```python
from build123d import *

# Parameters (mm, degrees)
SKETCH1_R             = 97.5
BOSS_EXTRUDE1_DEPTH   = 15
SKETCH2_R             = 27.5
CUT_EXTRUDE1_DEPTH    = 139.699315067
SKETCH3_R             = 3.589640567
CUT_EXTRUDE2_DEPTH    = 9.646154
CIRPATTERN1_START     = 5.353845626
CIRPATTERN1_OUTLINE_R = 3.589640567
CIRPATTERN1_DEPTH     = 9.646154374


# Read off the part's stored shape, not the designer's step: CirPattern1
with BuildPart() as part:
    # Sketch1 → Boss-Extrude1 (new body)
    with BuildSketch(Plane(origin=(0, 0, 0), x_dir=(1, 0, 0), z_dir=(0, 1, 0))):
        with Locations(Location((0, 0, 0), (0, 0, 270))):
            Circle(SKETCH1_R)
    extrude(amount=BOSS_EXTRUDE1_DEPTH)

    # Sketch2 → Cut-Extrude1 (cut, through all)
    with BuildSketch(Plane(origin=(0, 0, 0), x_dir=(1, 0, 0), z_dir=(0, 1, 0))):
        with Locations(Location((0, 0, 0), (0, 0, 270))):
            Circle(SKETCH2_R)
    extrude(amount=CUT_EXTRUDE1_DEPTH, mode=Mode.SUBTRACT)

    # Sketch3 → Cut-Extrude2 (cut)
    with BuildSketch(Plane(origin=(0, 15, 0), x_dir=(1, 0, 0), z_dir=(0, 1, 0))):
        with Locations(Location((-40.912084687, 0, 0), (0, 0, 270))):
            Circle(SKETCH3_R)
    extrude(amount=-CUT_EXTRUDE2_DEPTH, mode=Mode.SUBTRACT)

    # CirPattern1 outline → CirPattern1 (cut)
    with BuildSketch(Plane(origin=(0, 0, 0), x_dir=(1, 0, 0), z_dir=(0, 1, 0)).offset(CIRPATTERN1_START)):
        with Locations((0, 40.912084687)):
            Circle(CIRPATTERN1_OUTLINE_R)
        with Locations((40.912084687, 0)):
            Circle(CIRPATTERN1_OUTLINE_R)
        with Locations((0, -40.912084687)):
            Circle(CIRPATTERN1_OUTLINE_R)
    extrude(amount=CIRPATTERN1_DEPTH, mode=Mode.SUBTRACT)


solid = part.part
```
Check sheet for the modelled part. Datum: model origin and axes. Units: mm. A direction names the side the tool comes from. Give positions to 0.01 mm unless a question says otherwise; leave off trailing zeros. Order: outer loops, then holes, each group sorted by start corner. A loop starts at its lowest first (then second) coordinate and runs counter-clockwise, first axis right, second up. Notation, with made-up numbers: (49, 44.5) -> (76, 44.5) arc R23 cw to (76, 76.5) -> close; hole circle Ø4 at (-8.75, 62.25). An arc over 180 degrees is marked (long way). Return JSON: item names as keys, results as strings.
1. Mould release check, pull along Z, two halves, no side actions. Record for faces 3 (the cylindrical face through (-86.5, 7.4, 44.99)), 4 (the flat face through (-20, 15, 20)), 5 (the flat face through (-41, 5.354, 0)): +Z half, -Z half, draft (parallel to the pull), parting line (faces both ways), or undercut.
From the geometry:
{"face 3": "parting line", "face 4": "draft", "face 5": "undercut"}
2. Cross-section at C-C, the plane z = 52.5. Record the cut outline in (x, y), plus the area to 3 significant figures.
From the geometry:
{"outline": "(-82.16, 0) -> (82.16, 0) -> (82.16, 15) -> (-82.16, 15) -> close", "area": "2,460 mm^2"}
3. Cross-section at A-A, the plane x = 0. Record the cut outline in (y, z).
From the geometry:
{"outline": "(0, -97.5) -> (15, -97.5) -> (15, -44.5) -> (5.35, -44.5) -> (5.35, -37.32) -> (15, -37.32) -> (15, -27.5) -> (0, -27.5) -> close; (0, 27.5) -> (15, 27.5) -> (15, 37.32) -> (5.35, 37.32) -> (5.35, 44.5) -> (15, 44.5) -> (15, 97.5) -> (0, 97.5) -> close"}
4. Cross-section at B-B, the plane y = 11.75. Record the cut outline in (x, z).
From the geometry:
{"outline": "circle Ø195 at (0, 0); hole circle Ø7.18 at (-40.91, 0); hole circle Ø55 at (0, 0); hole circle Ø7.18 at (0, -40.91); hole circle Ø7.18 at (0, 40.91); hole circle Ø7.18 at (40.91, 0)"}
5. Cross-section at D-D, the plane x = 58.5. Record the cut outline in (y, z), plus the area to 3 significant figures.
From the geometry:
{"outline": "(0, -78) -> (15, -78) -> (15, 78) -> (0, 78) -> close", "area": "2,340 mm^2"}
6. Set-up check for faces 1 (the flat face through (0, 5.354, 41)), 2 (the flat face through (-20, 0, 20)): record each of +Z, -Z, +X, -X, +Y, -Y from which the full face is reachable in a straight line by a thin tool's end or side.
From the geometry:
{"face 1": "+Y", "face 2": "+Z, -Z, +X, -X, -Y"}
7. Material ranges on probe 1 along X at (y, z) = (11.25, 0); probe 2 along X at (y, z) = (12.75, -38); probe 3 along Z at (x, y) = (8.5, 12), recorded low to high. Write a range as [from, to].
From the geometry:
{"probe 1": "[-97.5, -44.5], [-37.32, -27.5], [27.5, 37.32], [44.5, 97.5]", "probe 2": "[-89.79, -2.1], [2.1, 89.79]", "probe 3": "[-97.13, -26.15], [26.15, 97.13]"}
8. Go/stop test with flat-tipped pins: P1, Ø3, axis at x = -54, y = 6, coming from the +Z side; P2, Ø5.5, axis at x = 40.91, z = 0, coming from the +Y side; P3, Ø3, axis at x = 12, y = 7, coming from the +Z side. Record where each tip stops, or that it passes through.
From the geometry:
{"P1": "z = 82.16", "P2": "y = 5.35", "P3": "z = 96.93"}
